from build123d import *

# Parameters (mm, degrees)
SKETCH1_R               = 55
SKETCH1_R_2             = 10
SKETCH1_W               = 20
SKETCH1_H               = 20
SKETCH1_W_2             = 10
SKETCH1_W_3             = 40
BOSS_EXTRUDE1_DEPTH     = 2.5
BOSS_EXTRUDE2_START     = 40
SKETCH2_R               = 55
SKETCH2_R_2             = 53.5
BOSS_EXTRUDE2_DEPTH     = 40
CUT_EXTRUDE1_START      = -5
SKETCH3_W               = 22
SKETCH3_H               = 22
SKETCH3_W_2             = 20
SKETCH3_H_2             = 20
SKETCH3_W_3             = 12
SKETCH3_W_4             = 10
SKETCH3_R               = 11
SKETCH3_R_2             = 10
CUT_EXTRUDE1_DEPTH      = 5
FILLET1_R               = 1
FILLET2_R               = 1
CUT_EXTRUDE2_DEPTH      = 88.464278486
CUT_EXTRUDE2_DEPTH_BACK = 88.464278486
SKETCH4_W               = 15
SKETCH4_H               = 5


with BuildPart() as part:
    # Sketch1 → Boss-Extrude1 (new body)
    # profile 1 of 2: a face of its own
    with BuildSketch(Plane(origin=(0, 0, 0), x_dir=(1, 0, 0), z_dir=(0, 1, 0))):
        with Locations(Location((0, 0, 0), (0, 0, 270))):
            Circle(SKETCH1_R)
        with Locations(Location((-40, -5, 0), (0, 0, 270))):
            Circle(SKETCH1_R_2, mode=Mode.SUBTRACT)
        with Locations((-20, 25)):
            Rectangle(SKETCH1_W, SKETCH1_H, mode=Mode.SUBTRACT)
        with Locations((-20, -5)):
            Rectangle(SKETCH1_W_2, SKETCH1_H, mode=Mode.SUBTRACT)
        Polygon((5, -15), (25, 5), (45, -15), align=None, mode=Mode.SUBTRACT)
        with Locations((0, -31.25)):
            Rectangle(SKETCH1_W_3, SKETCH1_H, mode=Mode.SUBTRACT)
        with BuildLine():
            Line((0, 15), (40, 15))
            ThreePointArc((40, 15), (20, 35), (0, 15))
        make_face(mode=Mode.SUBTRACT)
    # profile 2 of 2: a face of its own
    with BuildSketch(Plane(origin=(0, 0, 0), x_dir=(1, 0, 0), z_dir=(0, 1, 0))):
        with BuildLine():
            ThreePointArc((12.5, -41.25), (0, -28.75), (-12.5, -41.25))
            Line((-12.5, -41.25), (12.5, -41.25))
        make_face()
    extrude(amount=BOSS_EXTRUDE1_DEPTH)

    # Sketch2 → Boss-Extrude2 (add)
    with BuildSketch(Plane.XZ.offset(BOSS_EXTRUDE2_START)):
        with Locations(Location((0, 0, 0), (0, 0, 270))):
            Circle(SKETCH2_R)
        with Locations(Location((0, 0, 0), (0, 0, 270))):
            Circle(SKETCH2_R_2, mode=Mode.SUBTRACT)
    extrude(amount=-BOSS_EXTRUDE2_DEPTH)

    # Sketch3 → Cut-Extrude1 (cut)
    # profile 1 of 6: a face of its own
    with BuildSketch(Plane(origin=(0, 2.5, 0), x_dir=(1, 0, 0), z_dir=(0, 1, 0)).offset(CUT_EXTRUDE1_START)):
        with Locations((-20, 25)):
            Rectangle(SKETCH3_W, SKETCH3_H)
        with Locations((-20, 25)):
            Rectangle(SKETCH3_W_2, SKETCH3_H_2, mode=Mode.SUBTRACT)
    # profile 2 of 6: a face of its own
    with BuildSketch(Plane(origin=(0, 2.5, 0), x_dir=(1, 0, 0), z_dir=(0, 1, 0)).offset(CUT_EXTRUDE1_START)):
        with BuildLine():
            ThreePointArc((40.976176963, 14), (20, 36), (-0.976176963, 14))
            Line((-0.976176963, 14), (40.976176963, 14))
        make_face()
        with BuildLine():
            Line((40, 15), (0, 15))
            ThreePointArc((0, 15), (20, 35), (40, 15))
        make_face(mode=Mode.SUBTRACT)
    # profile 3 of 6: a face of its own
    with BuildSketch(Plane(origin=(0, 2.5, 0), x_dir=(1, 0, 0), z_dir=(0, 1, 0)).offset(CUT_EXTRUDE1_START)):
        with Locations((-20, -5)):
            Rectangle(SKETCH3_W_3, SKETCH3_H)
        with Locations((-20, -5)):
            Rectangle(SKETCH3_W_4, SKETCH3_H_2, mode=Mode.SUBTRACT)
    # profile 4 of 6: a face of its own
    with BuildSketch(Plane(origin=(0, 2.5, 0), x_dir=(1, 0, 0), z_dir=(0, 1, 0)).offset(CUT_EXTRUDE1_START)):
        Polygon((47.414213562, -16), (25, 6.414213562), (2.585786438, -16), align=None)
        Polygon((5, -15), (25, 5), (45, -15), align=None, mode=Mode.SUBTRACT)
    # profile 5 of 6: a face of its own
    with BuildSketch(Plane(origin=(0, 2.5, 0), x_dir=(1, 0, 0), z_dir=(0, 1, 0)).offset(CUT_EXTRUDE1_START)):
        with BuildLine():
            Line((21, -42.25), (21, -20.25))
            Line((21, -20.25), (-21, -20.25))
            Line((-21, -20.25), (-21, -42.25))
            Line((-21, -42.25), (-11.456439237, -42.25))
            ThreePointArc((-11.456439237, -42.25), (0, -29.75), (11.456439237, -42.25))
            Line((11.456439237, -42.25), (21, -42.25))
        make_face()
        with BuildLine():
            Line((-20, -21.25), (20, -21.25))
            Line((20, -21.25), (20, -41.25))
            Line((20, -41.25), (12.5, -41.25))
            ThreePointArc((12.5, -41.25), (0, -28.75), (-12.5, -41.25))
            Line((-12.5, -41.25), (-20, -41.25))
            Line((-20, -41.25), (-20, -21.25))
        make_face(mode=Mode.SUBTRACT)
    # profile 6 of 6: a face of its own
    with BuildSketch(Plane(origin=(0, 2.5, 0), x_dir=(1, 0, 0), z_dir=(0, 1, 0)).offset(CUT_EXTRUDE1_START)):
        with Locations(Location((-40, -5, 0), (0, 0, 270))):
            Circle(SKETCH3_R)
        with Locations((-40, -5)):
            Circle(SKETCH3_R_2, mode=Mode.SUBTRACT)
    extrude(amount=CUT_EXTRUDE1_DEPTH, mode=Mode.SUBTRACT)

    # Fillet1
    fillet1_edges = [part.edges().sort_by_distance(p)[0] for p in [
        (0, 2.5, -55),
    ]]
    fillet(fillet1_edges, radius=FILLET1_R)

    # Fillet2
    fillet2_edges = [part.edges().sort_by_distance(p)[0] for p in [
        (0, 0, 53.5),
    ]]
    fillet(fillet2_edges, radius=FILLET2_R)

    # Sketch4 → Cut-Extrude2 (cut, two sides: drawn at the far end of the back side and taken through both)
    with BuildSketch(Plane.XY.offset(-CUT_EXTRUDE2_DEPTH_BACK)):
        with Locations((0, -37.5)):
            Rectangle(SKETCH4_W, SKETCH4_H)
    extrude(amount=CUT_EXTRUDE2_DEPTH + CUT_EXTRUDE2_DEPTH_BACK, mode=Mode.SUBTRACT)


solid = part.part
Read the model definition and answer for the solid it produces. Units are mm, in the model's axes. A direction names the side the tool comes from. Give positions to 0.01 mm unless a question says otherwise; leave off trailing zeros. Write each loop counter-clockwise with the first axis right and the second up, starting at its lowest first coordinate (ties: lowest second). Pieces come first, ordered by that corner, then holes. Notation, with made-up numbers: M 72,0 L 89,0 A5 ccw 89,7 Z; hole C -38,89 d2. An arc over 180 degrees is marked long. One line per item, written item: value. Start each with the question number.
(1) Find section B-B (y = -25.5). Determine the outline of the cut face in (x, z).
(2) Find section A-A (z = 0). Determine the outline of the cut face in (x, y), plus the area to 3 significant figures.
(3) Find section C-C (z = -18). Give the number of separate pieces and of enclosed holes in the cut face, plus the area to 3 significant figures.
(4) Flat-ended cylindrical pins translate along their axes: pin 1 Ø3 at (y, z) = (1, -27) entering from +X; pin 2 Ø3 at (x, y) = (-21, 1.5) entering from -Z; pin 3 Ø1.2 at (x, y) = (-18, 1.5) entering from +Z. Find the tip coordinate at first contact, or state that the pin passes through.
(5) A tool of negligible diameter and unlimited length cuts with its end or side. For faces 4 (the flat face through (1, 0, -1)), 5 (the flat face through (-31, 1, -25)), from which of +Z, -Z, +X, -X, +Y, -Y can it reach the whole face along a straight path? Write none if from no direction.
(6) Determine the mould class of faces 1 (the flat face through (-21, 1, 31)), 2 (the flat face through (25, 1, 16)), 3 (the flat face through (54, -40, 4)) for opening direction Z: pulls with the +Z half, pulls with the -Z half, needs draft (parallel to the pull), parting line crosses it, or undercut.
(7) Find the intervals of material crossed by line 1 (X direction, y = -19, z = 0); line 2 (X direction, y = 1, z = 5), in increasing order.
Results below:
1. outline: C 0,0 d110; hole C 0,0 d107
2. outline: M -55,-40 L -53.5,-40 L -53.5,-1 A1 cw -52.5,0 L -49.8,0 L -49.8,2.5 L -54,2.5 A1 ccw -55,1.5 Z; M -30.2,0 L -26,0 L -26,2.5 L -30.2,2.5 Z; M -14,0 L 18.59,0 L 18.59,2.5 L -14,2.5 Z; M 31.41,0 L 52.5,0 A1 cw 53.5,-1 L 53.5,-40 L 55,-40 L 55,1.5 A1 ccw 54,2.5 L 31.41,2.5 Z
2. area: 284 mm^2
3. separate pieces: 3
3. enclosed holes: 0
3. area: 228 mm^2
4. pin 1: stops at x = 48.73
4. pin 2: stops at z = -51.43
4. pin 3: stops at z = 52.18
5. face 4: -Y
5. face 5: +Y, -Y
6. face 1: undercut
6. face 2: undercut
6. face 3: needs draft
7. line 1: x = -55 to -53.5, 53.5 to 55
7. line 2: x = -54.77 to -51, -29 to -26, -14 to 13.59, 36.41 to 54.77
